For this review, take the finished solid that the model builds, in its own axes (mm). Face numbers are marked on the shaded views. A direction names the side the tool comes from. Round coordinates to 2 decimals unless told otherwise and drop trailing zeros. Write each loop counter-clockwise with the first axis right and the second up, starting at its lowest first coordinate (ties: lowest second). Pieces come first, ordered by that corner, then holes. Notation, with made-up numbers: (1.25, -16.5) -> (27.25, -16.5) arc R10 cw to (27.25, -4.5) -> close; hole circle Ø9 at (62.5, 30.25). An arc over 180 degrees is marked (long way). Write each question's results on one line, items separated by ' | '. Start each with the question number.
Item 1: Add section C-C (y = 26). State the section outline as (x, z) points.
Item 2: Clearance check with flat-ended pins moving along their axes: pin 1 (2.5 mm diameter, centred on x = -53.5, y = 6, fed in from +Z); pin 2 (2.5 mm diameter, centred on x = -47.65, y = 4, fed in from -Z); pin 3 (7 mm diameter, centred on x = -55, y = 44, fed in from -Z). State where each tip first meets the part, or that it passes through.
Item 3: Add section B-B (z = 4). Count the separate pieces of the cut face and the enclosed holes in it, plus the area to 3 significant figures.
Item 4: The part is to be moulded in two halves that separate along X. For the marked faces 1, 2, 3 and 4, say which applies: +X half, -X half, draft (parallel to the pull), parting line (faces both ways), or undercut.
Item 5: To check wall thickness, follow line 1 along Y through (x, z) = (-55, 2); line 2 along Y through (x, z) = (-55, 7); line 3 along Y through (x, z) = (-40, 5.5). State the ranges of each line that lie inside material, in increasing order.
Item 6: Tool access review of the marked faces 5 and 6: name each direction out of +Z, -Z, +X, -X, +Y, -Y from which nothing blocks a thin tool from reaching the whole face with its end or side.
Item 7: Add section A-A (x = -40). State the section outline as (y, z) points.
from build123d import *

# Parameters (mm, degrees)
SKETCH1_W           = 60
SKETCH1_H           = 50
SKETCH1_R           = 4
SKETCH1_R_2         = 2.25
SKETCH1_R_3         = 2.75
SKETCH1_R_4         = 2
BOSS_EXTRUDE2_DEPTH = 10
SKETCH2_R           = 4
CUT_EXTRUDE1_DEPTH  = 4
SKETCH3_R           = 5
CUT_EXTRUDE2_DEPTH  = 5


with BuildPart() as part:
    # Sketch1 → Boss-Extrude2 (new body)
    with BuildSketch(Plane.XY):
        with Locations((-30, 25)):
            Rectangle(SKETCH1_W, SKETCH1_H)
        with Locations((-10, 41)):
            Circle(SKETCH1_R, mode=Mode.SUBTRACT)
        with Locations((-10, 9)):
            Circle(SKETCH1_R, mode=Mode.SUBTRACT)
        with Locations((-40, 9)):
            Circle(SKETCH1_R, mode=Mode.SUBTRACT)
        with Locations((-40, 41)):
            Circle(SKETCH1_R, mode=Mode.SUBTRACT)
        with Locations((-55, 44)):
            Circle(SKETCH1_R_2, mode=Mode.SUBTRACT)
        with Locations((-55, 6)):
            Circle(SKETCH1_R_2, mode=Mode.SUBTRACT)
        with Locations((-44, 25)):
            Circle(SKETCH1_R_3, mode=Mode.SUBTRACT)
        with Locations((-6, 25)):
            Circle(SKETCH1_R_3, mode=Mode.SUBTRACT)
        with Locations((-47.652499067, 46)):
            Circle(SKETCH1_R_4, mode=Mode.SUBTRACT)
        with Locations((-47.652499067, 4)):
            Circle(SKETCH1_R_4, mode=Mode.SUBTRACT)
    extrude(amount=BOSS_EXTRUDE2_DEPTH)

    # Sketch2 → Cut-Extrude1 (cut)
    with BuildSketch(Plane.XY.offset(10)):
        with Locations((-55, 44)):
            Circle(SKETCH2_R)
        with Locations((-55, 6)):
            Circle(SKETCH2_R)
    extrude(amount=-CUT_EXTRUDE1_DEPTH, mode=Mode.SUBTRACT)

    # Sketch3 → Cut-Extrude2 (cut)
    with BuildSketch(Plane.XY.offset(10)):
        with Locations((-44, 25)):
            Circle(SKETCH3_R)
        with Locations((-6, 25)):
            Circle(SKETCH3_R)
    extrude(amount=-CUT_EXTRUDE2_DEPTH, mode=Mode.SUBTRACT)


solid = part.part
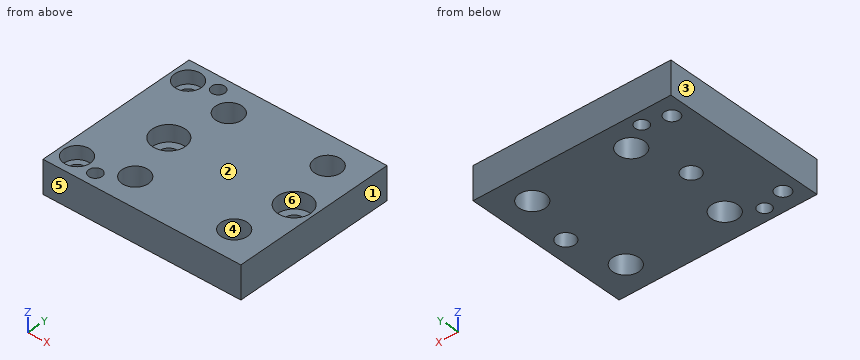
Responses:
1) outline: (-60, 0) -> (-46.56, 0) -> (-46.56, 5) -> (-48.9, 5) -> (-48.9, 10) -> (-60, 10) -> close; (-41.44, 0) -> (-8.56, 0) -> (-8.56, 5) -> (-10.9, 5) -> (-10.9, 10) -> (-39.1, 10) -> (-39.1, 5) -> (-41.44, 5) -> close; (-3.44, 0) -> (0, 0) -> (0, 10) -> (-1.1, 10) -> (-1.1, 5) -> (-3.44, 5) -> close
2) pin 1: stops at z = 6 | pin 2: passes through | pin 3: stops at z = 0
3) separate pieces: 1 | enclosed holes: 10 | area: 2,690 mm^2
4) face 1: +X half | face 2: draft | face 3: -X half | face 4: undercut
5) line 1: y = 0 to 3.75, 8.25 to 41.75, 46.25 to 50 | line 2: y = 0 to 2, 10 to 40, 48 to 50 | line 3: y = 0 to 5, 13 to 22, 28 to 37, 45 to 50
6) face 5: +Z, -Z, +X, -X, -Y | face 6: +Z
7) outline: (0, 0) -> (5, 0) -> (5, 10) -> (0, 10) -> close; (13, 0) -> (37, 0) -> (37, 10) -> (28, 10) -> (28, 5) -> (22, 5) -> (22, 10) -> (13, 10) -> close; (45, 0) -> (50, 0) -> (50, 10) -> (45, 10) -> close
